Verification items for the finished model (mm, model axes). A direction names the side the tool comes from. Round coordinates to 2 decimals unless told otherwise and drop trailing zeros. Write each loop counter-clockwise with the first axis right and the second up, starting at its lowest first coordinate (ties: lowest second). Pieces come first, ordered by that corner, then holes. Notation, with made-up numbers: (58, -11) - (83, -11) arc R25 ccw to (83, 15) - close; hole circle Ø1 at (82.5, -10.75). An arc over 180 degrees is marked (long way). Answer as a JSON object with one key per item and string values. Group by question number.
1) Section check B-B (x = 21). Enter the section's corners in (y, z).
2) Section check A-A (y = 5). Enter the section's corners in (x, z).
3) Thickness scan on line 1 (Y direction, x = 12.8, z = 4.1); line 2 (X direction, y = 20.5, z = 2.1); line 3 (X direction, y = -14, z = 3.65). Record the ranges inside material, lowest first.
4) Mould release check, pull along Y, two halves, no side actions. Record for faces 1 (the flat face through (41, -2, 3)), 2 (the cylindrical face through (40.4, -24.18, 2.96)), 3 (the flat face through (-35.08, 8.14, 2.96)), 4 (the cylindrical face through (39.241, 22.895, 2.958)): +Y half, -Y half, draft (parallel to the pull), parting line (faces both ways), or undercut.
5) Section check C-C (x = -20.5). Enter the section's corners in (y, z).
6) Set-up check for faces 5 (the flat face through (-6.61, 10.33, 2.96)), 6 (the flat face through (-41, 0, 3)): record each of +Z, -Z, +X, -X, +Y, -Y from which the full face is reachable in a straight line by a thin tool's end or side.
7) Section check D-D (y = -5). Enter the section's corners in (x, z).
```python
from build123d import *

# Parameters (mm, degrees)
F0_R     = 12.5
F0_R_2   = 2.55
F0_R_3   = 1.3
F0_R_4   = 1.6
F1_DEPTH = 6


# Not quite as in the source:
# - ends of sketch curves that miss each other by under 0.0002 mm in the source are joined


with BuildPart() as f1:
    # F0 (on Top) → F1 (new body)
    with BuildSketch(Plane.XY):
        with BuildLine():
            Line((34.83, 24.75), (-34.83, 24.75))
            ThreePointArc((-34.83, 24.75), (-39.1928488399, 22.9428488399), (-41, 18.58))
            Line((-41, 18.58), (-41, -18.58))
            ThreePointArc((-41, -18.58), (-39.1928488399, -22.9428488399), (-34.83, -24.75))
            Line((-34.83, -24.75), (39, -24.75))
            ThreePointArc((39, -24.75), (40.4142135624, -24.1642135624), (41, -22.75))
            Line((41, -22.75), (41, 18.58))
            ThreePointArc((41, 18.58), (39.1928488399, 22.9428488399), (34.83, 24.75))
        make_face()
        with BuildLine():
            ThreePointArc((-34.1539839892, -21.5960150108), (-36.3460155108, -21.5960155108), (-36.3460150108, -19.4039839892))
            Line((-36.346015, -19.403984), (-33.846015, -16.903984))
            ThreePointArc((-33.8460150108, -16.9039839892), (-31.6539844892, -16.9039844892), (-31.6539839892, -19.0960150108))
            Line((-31.653984, -19.096015), (-34.153984, -21.596015))
        make_face(mode=Mode.SUBTRACT)
        with BuildLine():
            ThreePointArc((-3.1539844892, -19.4039844892), (-3.1539844892, -21.5960155108), (-5.3460155108, -21.5960155108))
            Line((-5.3460155108, -21.5960155108), (-7.846015, -19.096015))
            ThreePointArc((-7.846015, -19.096015), (-7.8460155108, -16.9039844892), (-5.6539844892, -16.9039844892))
            Line((-5.6539844892, -16.9039844892), (-3.1539844892, -19.4039844892))
        make_face(mode=Mode.SUBTRACT)
        with Locations((-19.25, -5)):
            Circle(F0_R, mode=Mode.SUBTRACT)
        with Locations((12.8, -15)):
            Circle(F0_R_2, mode=Mode.SUBTRACT)
        with Locations((36.4, -21.75)):
            Circle(F0_R_3, mode=Mode.SUBTRACT)
        with Locations((32.8, -15)):
            Circle(F0_R_2, mode=Mode.SUBTRACT)
        with Locations((12.8, -5)):
            Circle(F0_R_2, mode=Mode.SUBTRACT)
        with Locations((32.8, -5)):
            Circle(F0_R_2, mode=Mode.SUBTRACT)
        with BuildLine():
            ThreePointArc((-31.6539844892, 9.0960155108), (-31.6539844892, 6.9039844892), (-33.8460155108, 6.9039844892))
            Line((-33.8460155108, 6.9039844892), (-36.346015, 9.403985))
            ThreePointArc((-36.346015, 9.403985), (-36.3460155108, 11.5960155108), (-34.1539844892, 11.5960155108))
            Line((-34.1539844892, 11.5960155108), (-31.6539844892, 9.0960155108))
        make_face(mode=Mode.SUBTRACT)
        with BuildLine():
            ThreePointArc((-5.3460150108, 11.5960160108), (-3.1539844892, 11.5960155108), (-3.1539839892, 9.4039849892))
            Line((-3.153984, 9.403985), (-5.653984, 6.903985))
            ThreePointArc((-5.6539839892, 6.9039849892), (-7.8460155108, 6.9039844892), (-7.8460150108, 9.0960160108))
            Line((-7.846015, 9.096016), (-5.346015, 11.596016))
        make_face(mode=Mode.SUBTRACT)
        with Locations((-21, 19.75)):
            Circle(F0_R_4, mode=Mode.SUBTRACT)
        with Locations((12.8, 5)):
            Circle(F0_R_2, mode=Mode.SUBTRACT)
        with Locations((32.8, 5)):
            Circle(F0_R_2, mode=Mode.SUBTRACT)
        with Locations((0, 19.75)):
            Circle(F0_R_4, mode=Mode.SUBTRACT)
        with Locations((21, 19.75)):
            Circle(F0_R_4, mode=Mode.SUBTRACT)
    extrude(amount=F1_DEPTH)


solid = f1.part
```
Returned:
{
 "1": {"outline": "(-24.75, 0) - (18.15, 0) - (18.15, 6) - (-24.75, 6) - close; (21.35, 0) - (24.75, 0) - (24.75, 6) - (21.35, 6) - close"},
 "2": {"outline": "(-41, 0) - (-26.75, 0) - (-26.75, 6) - (-41, 6) - close; (-11.75, 0) - (10.25, 0) - (10.25, 6) - (-11.75, 6) - close; (15.35, 0) - (30.25, 0) - (30.25, 6) - (15.35, 6) - close; (35.35, 0) - (41, 0) - (41, 6) - (35.35, 6) - close"},
 "3": {"line 1": "-24.75 to -17.55, -12.45 to -7.55, -2.45 to 2.45, 7.55 to 24.75", "line 2": "-40.69 to -22.41, -19.59 to -1.41, 1.41 to 19.59, 22.41 to 40.69", "line 3": "-41 to -27.92, -10.58 to 10.45, 15.15 to 30.45, 35.15 to 41"},
 "4": {"face 1": "draft", "face 2": "-Y half", "face 3": "undercut", "face 4": "+Y half"},
 "5": {"outline": "(-24.75, 0) - (-17.44, 0) - (-17.44, 6) - (-24.75, 6) - close; (7.44, 0) - (18.23, 0) - (18.23, 6) - (7.44, 6) - close; (21.27, 0) - (24.75, 0) - (24.75, 6) - (21.27, 6) - close"},
 "6": {"face 5": "+Z, -Z", "face 6": "+Z, -Z, -X, +Y, -Y"},
 "7": {"outline": "(-41, 0) - (-31.75, 0) - (-31.75, 6) - (-41, 6) - close; (-6.75, 0) - (10.25, 0) - (10.25, 6) - (-6.75, 6) - close; (15.35, 0) - (30.25, 0) - (30.25, 6) - (15.35, 6) - close; (35.35, 0) - (41, 0) - (41, 6) - (35.35, 6) - close"}
}
